```python
from build123d import *

# Parameters (mm, degrees)
SKETCH1_R           = 12
BOSS_EXTRUDE1_DEPTH = 18.6875
SKETCH1_4_R         = 12
BOSS_EXTRUDE2_DEPTH = 57.5


with BuildPart() as part:
    # Sketch1 → Boss-Extrude1 (new body, symmetric)
    with BuildSketch(Plane.XY):
        with BuildLine():
            Line((125, 80.499531502), (125, -137.375))
            ThreePointArc((125, -137.375), (0, -262.375), (-125, -137.375))
            Line((-125, -137.375), (-125, 80.5))
            Line((-125, 80.5), (-89.72361368, 122.703318674))
            Line((-89.72361368, 122.703318674), (89.723613553, 122.703318674))
            Line((89.723613553, 122.703318674), (125, 80.499531502))
        make_face()
        with Locations((0, 37.375)):
            Circle(SKETCH1_R, mode=Mode.SUBTRACT)
        with Locations((0, -137.375)):
            Circle(SKETCH1_R, mode=Mode.SUBTRACT)
    extrude(amount=BOSS_EXTRUDE1_DEPTH, both=True)

    # Sketch1_4 → Boss-Extrude2 (add)
    with BuildSketch(Plane.XY):
        with Locations((0, -50)):
            Circle(SKETCH1_4_R)
    extrude(amount=BOSS_EXTRUDE2_DEPTH)


solid = part.part
```
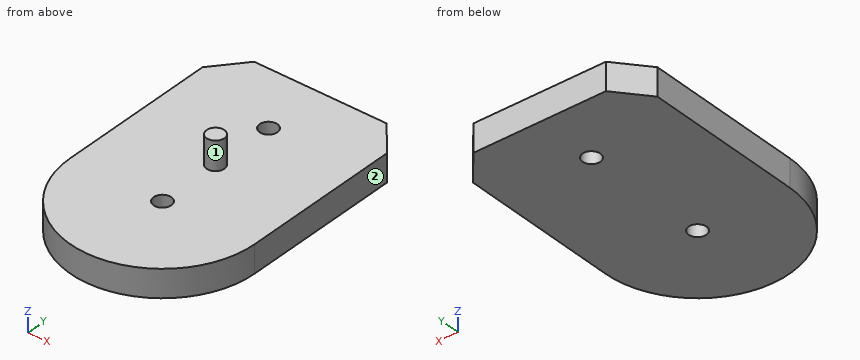
Geometry: final body of the model. Coordinates: model frame, mm. Face numbers are marked on the shaded views. A direction names the side the tool comes from. Coordinates: 2 decimals unless noted, no trailing zeros. Order: outer loops, then holes, each group sorted by start corner. A loop starts at its lowest first (then second) coordinate and runs counter-clockwise, first axis right, second up. Notation, with made-up numbers: (-2, 73) - (27, 73) arc R15 ccw to (27, 102) - close; hole circle Ø2 at (75.25, 41.5). An arc over 180 degrees is marked (long way). Write each question's results on one line, items separated by ' | '.
(1) Section query D-D, the plane z = 29. Return the cut outline in (x, y).
Values found:
outline: circle Ø24 at (0, -50)
(2) Section query B-B, the plane y = -50. Return the cut outline in (x, z).
Values found:
outline: (-125, -18.69) - (125, -18.69) - (125, 18.69) - (12, 18.69) - (12, 57.5) - (-12, 57.5) - (-12, 18.69) - (-125, 18.69) - close
(3) Section query C-C, the plane z = -13. Return the cut outline in (x, y) (3 decimals), plus the area to 3 significant figures.
Values found:
outline: (-125, -137.375) arc R125 ccw to (125, -137.375) - (125, 80.5) - (89.724, 122.703) - (-89.724, 122.703) - (-125, 80.5) - close; hole circle Ø24 at (0, -137.375); hole circle Ø24 at (0, 37.375) | area: 87,200 mm²
(4) Set-up query: the marked faces 1 and 2. Return all of +Z, -Z, +X, -X, +Y, -Y with unobstructed straight access to the full face (end or side cutting, diameter ignored); none if empty.
Values found:
face 1: +Z | face 2: +Z, -Z, +X, +Y, -Y
(5) Section query A-A, the plane x = 0. Return the cut outline in (y, z) (1 decimal), plus the area to 3 significant figures.
Values found:
outline: (-262.4, -18.7) - (-149.4, -18.7) - (-149.4, 18.7) - (-262.4, 18.7) - close; (-125.4, -18.7) - (25.4, -18.7) - (25.4, 18.7) - (-38, 18.7) - (-38, 57.5) - (-62, 57.5) - (-62, 18.7) - (-125.4, 18.7) - close; (49.4, -18.7) - (122.7, -18.7) - (122.7, 18.7) - (49.4, 18.7) - close | area: 13,500 mm²
(6) Line query: line 1 (Y direction, x = 0, z = 1) (3 decimals); line 2 (Z direction, x = 40.5, y = -72); line 3 (Y direction, x = 26, z = -4.5). Output: solid intervals per line, ascending. Write a range as [from, to].
Values found:
line 1: y = [-262.375, -149.375], [-125.375, 25.375], [49.375, 122.703] | line 2: z = [-18.69, 18.69] | line 3: y = [-259.64, 122.7]
(7) First-contact query: pin 1 Ø5 at (x, z) = (96.5, 12) entering from +Y; pin 2 Ø12 at (y, z) = (-188, 0) entering from +X; pin 3 Ø8 at (x, y) = (-47, -108.5) entering from +Z; pin 4 Ø14.5 at (x, y) = (0, -137.375) entering from -Z. Flat tips, straight axial feed; report the tip coordinate or a pass-through.
Values found:
pin 1: stops at y = 117.59 | pin 2: stops at x = 116.76 | pin 3: stops at z = 18.69 | pin 4: passes through
